Verification items for the finished model (mm, model axes). Face numbers are marked on the shaded views. A direction names the side the tool comes from. Round coordinates to 2 decimals unless told otherwise and drop trailing zeros. Write each loop counter-clockwise with the first axis right and the second up, starting at its lowest first coordinate (ties: lowest second). Pieces come first, ordered by that corner, then holes. Notation, with made-up numbers: M 49,-9.5 L 56,-9.5 A28 ccw 56,14.5 Z; hole C 29,29.25 d5. An arc over 180 degrees is marked long. Answer in a Markdown table with one row per item. Add a question column.
1. Set-up check for the marked faces 1, 2, 3 and 4: record each of +Z, -Z, +X, -X, +Y, -Y from which the full face is reachable in a straight line by a thin tool's end or side.
2. Sectioned sample at A-A on z = -14. Record the cut outline in (x, y), plus the area to 3 significant figures.
3. Draft check along Z on the marked faces 5, 6 and 7. Enter one of: pulls with the +Z half, pulls with the -Z half, needs draft (parallel to the pull), parting line crosses it, or undercut.
4. Sectioned sample at D-D on z = -20. Record the cut outline in (x, y).
5. Sectioned sample at B-B on y = 0. Record the cut outline in (x, z), plus the area to 3 significant figures.
6. Material ranges on probe 1 along Y at (x, z) = (-2, -23.5); probe 2 along X at (y, z) = (2.55, -20); probe 3 along Z at (x, y) = (0, -3.4), recorded low to high.
7. Sectioned sample at C-C on x = 0. Count the separate pieces of the cut face and the enclosed holes in it, plus the area to 3 significant figures.
8. Go/stop test with flat-tipped pins: pin 1 Ø4 at (x, z) = (2.5, -18.5) entering from -Y; pin 2 Ø6 at (x, z) = (0, 23) entering from +Y; pin 3 Ø3 at (x, z) = (0, -20) entering from +Y; pin 4 Ø3.5 at (x, y) = (1, 0) entering from +Z. Record where each tip stops, or that it passes through.
Autodesk Inventor part; units mm, degrees
ref_plane "YZ Plane" through (0, 0, 0) normal (1, 0, 0) x (0, 1, 0)
ref_plane "XZ Plane" through (0, 0, 0) normal (0, 1, 0) x (-1, 0, 0)
ref_plane "XY Plane" through (0, 0, 0) normal (0, 0, 1) x (1, 0, 0)
sketch "Esboço1" plane through (0, 0, 0) normal (1, 0, 0) x (0, 1, 0)
  circle A0 centre (0, 0) radius 11
  line L0 (1.5, -27.5) -> (1.5, -12.4097)
  line L1 (1.5, 12.4097) -> (1.5, 27.5)
  line L2 (4.5, -27.5) -> (4.5, -11.6619)
  line L3 (4.5, 11.6619) -> (4.5, 27.5)
  line L4 (-4.5, 27.5) -> (-4.5, 11.6619)
  line L5 (-4.5, -11.6619) -> (-4.5, -27.5)
  line L6 (-1.5, 27.5) -> (-1.5, 12.4097)
  line L7 (-1.5, -12.4097) -> (-1.5, -27.5)
  line L8 (-4.5, -27.5) -> (-1.5, -27.5)
  line L9 (1.5, -27.5) -> (4.5, -27.5)
  line L10 (4.5, 27.5) -> (1.5, 27.5)
  line L11 (-1.5, 27.5) -> (-4.5, 27.5)
  line L12 (0, -12.5) -> (1.5, -12.5)
  line L13 (0, -12.5) -> (-1.5, -12.5)
  line L14 (0, 12.5) -> (1.5, 12.5)
  line L15 (0, 12.5) -> (-1.5, 12.5)
  arc A1 (-1.5, 12.4097) -> (-1.5, -12.4097) centre (0, 0) ccw
  arc A2 (1.5, -12.4097) -> (1.5, 12.4097) centre (0, 0) ccw
  dimension "d0" = 22
extrude "Extrusão1" add sketch "Esboço1" along normal mid plane 12
sketch "Esboço2" plane through (-6, 4.5, 27.5) normal (0, 1, 0) x (1, 0, 0)
  point P0 (6, 27.5)
sketch "Esboço3" plane through (-6, -1.5, 27.5) normal (0, 1, 0) x (1, 0, 0)
  circle A0 centre (6, 7.5) radius 2.5
  line L0 (0, 0) -> (12, 0)
  line L1 (12, 15) -> (12, 0)
  line L2 (0, 0) -> (0, 15.8381)
  point P0 (6, 27.5)
  dimension "d17" = 5
  dimension "d18" = 7.5
  dimension "d19" = 6
hole "Furo1" at (0, -1.5, 20) direction (0, -1, 0) diameter 5 end through all both
sketch "Esboço4" plane through (-6, -1.5, -12.5) normal (0, 1, 0) x (1, 0, 0)
  circle A0 centre (6, 7.5) radius 2.5
  line L0 (12, 15) -> (0, 15)
  line L1 (12, 15) -> (12, -0.8381)
  point P0 (6, -12.5)
  dimension "d28" = 5
  dimension "d29" = 7.5
  dimension "d30" = 6
hole "Furo2" at (0, -1.5, -20) direction (0, -1, 0) diameter 5 end through all both
fillet "Arredondamento1" radius 2 12 edges at (0, 4.5, 11.6619) (0, 4.5, -11.6619) (0, -4.5, -11.6619) (0, -4.5, 11.6619) (6, 3, 27.5) (-6, 3, 27.5) (-6, -3, 27.5) (6, -3, 27.5) (6, 3, -27.5) (6, -3, -27.5) (-6, -3, -27.5) (-6, 3, -27.5)
properties part number "Abraçadeira_CPY1_CPY_CPY1" material "ABS plástico"
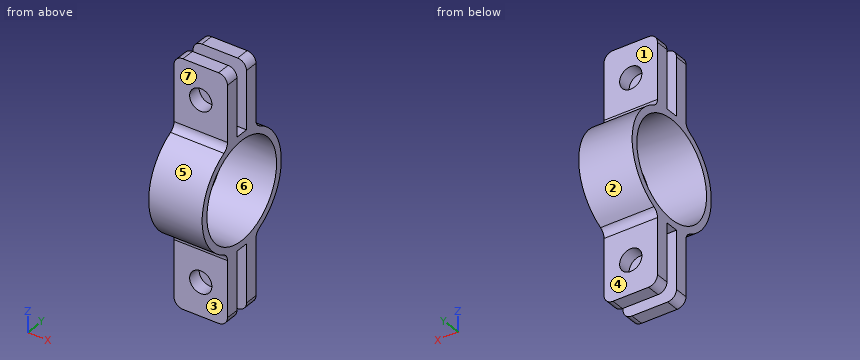
Geometry check:
| question | item | result |
|---|---|---|
| 1 | face 1 | +Z, +X, -X, +Y |
| 1 | face 2 | +X, -X, +Y |
| 1 | face 3 | -Z, +X, -X, -Y |
| 1 | face 4 | -Z, +X, -X, +Y |
| 2 | outline | M -6,-4.5 L 6,-4.5 L 6,-1.5 L -6,-1.5 Z; M -6,1.5 L 6,1.5 L 6,4.5 L -6,4.5 Z |
| 2 | area | 72.0 mm2 |
| 3 | face 5 | parting line crosses it |
| 3 | face 6 | undercut |
| 3 | face 7 | needs draft |
| 4 | outline | M -6,-4.5 L -2.5,-4.5 L -2.5,-1.5 L -6,-1.5 Z; M -6,1.5 L -2.5,1.5 L -2.5,4.5 L -6,4.5 Z; M 2.5,-4.5 L 6,-4.5 L 6,-1.5 L 2.5,-1.5 Z; M 2.5,1.5 L 6,1.5 L 6,4.5 L 2.5,4.5 Z |
| 5 | outline | M -6,-12.5 L 6,-12.5 L 6,-11 L -6,-11 Z; M -6,11 L 6,11 L 6,12.5 L -6,12.5 Z |
| 5 | area | 36.0 mm2 |
| 6 | probe 1 | y = -4.5 to -1.5, 1.5 to 4.5 |
| 6 | probe 2 | x = -6 to -2.5, 2.5 to 6 |
| 6 | probe 3 | z = -27.5 to -22.5, -17.5 to -10.46, 10.46 to 17.5, 22.5 to 27.5 |
| 7 | separate pieces | 5 |
| 7 | enclosed holes | 1 |
| 7 | area | 237 mm2 |
| 8 | pin 1 | stops at y = -4.5 |
| 8 | pin 2 | stops at y = 4.5 |
| 8 | pin 3 | passes through |
| 8 | pin 4 | stops at z = 27.5 |
